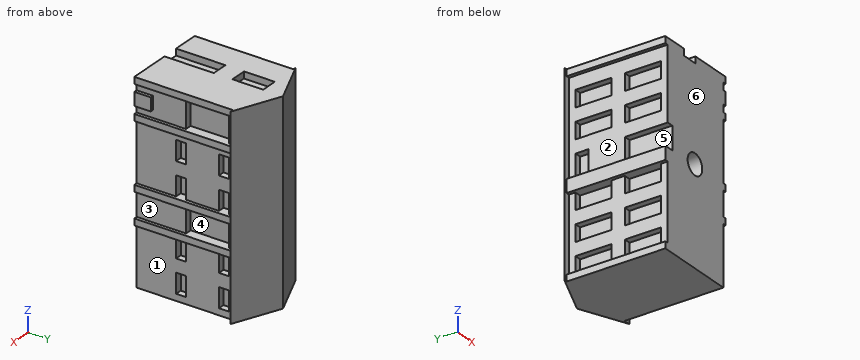
```python
from build123d import *

# Parameters (mm, degrees)
SALIENTE_EXTRUIR1_DEPTH = 30
CROQUIS2_W              = 1
CROQUIS2_H              = 15
SALIENTE_EXTRUIR2_DEPTH = 0.5
CROQUIS3_W              = 1
CROQUIS3_H              = 15
SALIENTE_EXTRUIR3_DEPTH = 0.5
CROQUIS3_3_W            = 3
CROQUIS3_3_H            = 1.5
CROQUIS3_3_W_2          = 3.754100145
CROQUIS3_3_H_2          = 6.5
CROQUIS3_3_W_3          = 4.245899855
CORTAR_EXTRUIR1_DEPTH   = 1
CROQUIS3_4_W            = 2
CROQUIS3_4_H            = 2.5
SALIENTE_EXTRUIR4_DEPTH = 0.5
CROQUIS7_W              = 1
CROQUIS7_H              = 15
SALIENTE_EXTRUIR5_DEPTH = 0.5
CROQUIS8_W              = 2.5
CROQUIS8_H              = 7.5
CROQUIS8_H_2            = 4.684108695
CORTAR_EXTRUIR2_DEPTH   = 1
CROQUIS10_W             = 1
CROQUIS10_H             = 15
CROQUIS10_W_2           = 2
SALIENTE_EXTRUIR6_DEPTH = 0.5
CROQUIS11_W             = 2.5
CROQUIS11_H             = 5.5
CORTAR_EXTRUIR3_DEPTH   = 1
CROQUIS12_W             = 3.5
CROQUIS12_H             = 6.5
CROQUIS12_H_2           = 2
CROQUIS12_W_2           = 2.5
CROQUIS12_H_3           = 5.5
CORTAR_EXTRUIR4_DEPTH   = 1
CROQUIS13_R             = 1.575
CORTAR_EXTRUIR5_DEPTH   = 2.5


with BuildPart() as part:
    # Croquis1 → Saliente-Extruir1 (new body)
    with BuildSketch(Plane.XY):
        Polygon((-6, -7.5), (6, -7.5), (6, 7.5), (7, 7.5), (0, 10.5), (-7, 7.5), (-6, 7.5), align=None)
    extrude(amount=SALIENTE_EXTRUIR1_DEPTH)

    # Croquis2 → Saliente-Extruir2 (add)
    with BuildSketch(Plane(origin=(6, 0, 0), x_dir=(0, 0, -1), z_dir=(1, 0, 0))):
        with Locations((-29.5, 0)):
            Rectangle(CROQUIS2_W, CROQUIS2_H)
        with Locations((-24.254100145, 0)):
            Rectangle(CROQUIS2_W, CROQUIS2_H)
    extrude(amount=SALIENTE_EXTRUIR2_DEPTH)

    # Croquis3 → Saliente-Extruir3 (add)
    with BuildSketch(Plane(origin=(6, 0, 0), x_dir=(0, 0, -1), z_dir=(1, 0, 0))):
        with Locations((-14.254100145, 0)):
            Rectangle(CROQUIS3_W, CROQUIS3_H)
        with Locations((-9.5, 0)):
            Rectangle(CROQUIS3_W, CROQUIS3_H)
    extrude(amount=SALIENTE_EXTRUIR3_DEPTH)

    # Croquis3_3 → Cortar-Extruir1 (cut)
    with BuildSketch(Plane(origin=(6, 0, 0), x_dir=(0, 0, -1), z_dir=(1, 0, 0))):
        with Locations((-21.254100145, 5.75)):
            Rectangle(CROQUIS3_3_W, CROQUIS3_3_H)
        with Locations((-16.254100145, 5.75)):
            Rectangle(CROQUIS3_3_W, CROQUIS3_3_H)
        with Locations((-16.254100145, -0.75)):
            Rectangle(CROQUIS3_3_W, CROQUIS3_3_H)
        with Locations((-21.254100145, -0.75)):
            Rectangle(CROQUIS3_3_W, CROQUIS3_3_H)
        with Locations((-7.5, -0.75)):
            Rectangle(CROQUIS3_3_W, CROQUIS3_3_H)
        with Locations((-2.5, -0.75)):
            Rectangle(CROQUIS3_3_W, CROQUIS3_3_H)
        with Locations((-11.877050073, 3.25)):
            Rectangle(CROQUIS3_3_W_2, CROQUIS3_3_H_2)
        with Locations((-7.5, 5.75)):
            Rectangle(CROQUIS3_3_W, CROQUIS3_3_H)
        with Locations((-2.5, 5.75)):
            Rectangle(CROQUIS3_3_W, CROQUIS3_3_H)
        with Locations((-26.877050073, 3.25)):
            Rectangle(CROQUIS3_3_W_3, CROQUIS3_3_H_2)
    extrude(amount=-CORTAR_EXTRUIR1_DEPTH, mode=Mode.SUBTRACT)

    # Croquis3_4 → Saliente-Extruir4 (add)
    with BuildSketch(Plane(origin=(6, 0, 0), x_dir=(0, 0, -1), z_dir=(1, 0, 0))):
        with Locations((-26.877050072, -6.25)):
            Rectangle(CROQUIS3_4_W, CROQUIS3_4_H)
    extrude(amount=SALIENTE_EXTRUIR4_DEPTH)

    # Croquis7 → Saliente-Extruir5 (add)
    with BuildSketch(Plane.ZY.offset(6)):
        with Locations((29.5, 0)):
            Rectangle(CROQUIS7_W, CROQUIS7_H)
    extrude(amount=SALIENTE_EXTRUIR5_DEPTH)

    # Croquis8 → Cortar-Extruir2 (cut)
    with BuildSketch(Plane.XY.offset(30)):
        with Locations((-1.25, -3.75)):
            Rectangle(CROQUIS8_W, CROQUIS8_H)
        with Locations((-1.25, 5.157945653)):
            Rectangle(CROQUIS8_W, CROQUIS8_H_2)
    extrude(amount=-CORTAR_EXTRUIR2_DEPTH, mode=Mode.SUBTRACT)

    # Croquis10 → Saliente-Extruir6 (add)
    with BuildSketch(Plane.ZY.offset(6)):
        with Locations((0.5, 0)):
            Rectangle(CROQUIS10_W, CROQUIS10_H)
        with Locations((13.5, 0)):
            Rectangle(CROQUIS10_W_2, CROQUIS10_H)
    extrude(amount=SALIENTE_EXTRUIR6_DEPTH)

    # Croquis11 → Cortar-Extruir3 (cut)
    with BuildSketch(Plane.ZY.offset(6)):
        with Locations((6.75, 3.75)):
            Rectangle(CROQUIS11_W, CROQUIS11_H)
        with Locations((2.25, 3.75)):
            Rectangle(CROQUIS11_W, CROQUIS11_H)
        with Locations((11.25, 3.75)):
            Rectangle(CROQUIS11_W, CROQUIS11_H)
        with Locations((6.75, -3.75)):
            Rectangle(CROQUIS11_W, CROQUIS11_H)
        with Locations((11.25, -3.75)):
            Rectangle(CROQUIS11_W, CROQUIS11_H)
        with Locations((2.25, -3.75)):
            Rectangle(CROQUIS11_W, CROQUIS11_H)
    extrude(amount=-CORTAR_EXTRUIR3_DEPTH, mode=Mode.SUBTRACT)

    # Croquis12 → Cortar-Extruir4 (cut)
    with BuildSketch(Plane.ZY.offset(6)):
        with Locations((16.25, -4.25)):
            Rectangle(CROQUIS12_W, CROQUIS12_H)
        with Locations((16.25, 5.5)):
            Rectangle(CROQUIS12_W, CROQUIS12_H_2)
        with Locations((21.25, 3.75)):
            Rectangle(CROQUIS12_W_2, CROQUIS12_H_3)
        with Locations((25.75, 3.75)):
            Rectangle(CROQUIS12_W_2, CROQUIS12_H_3)
        with Locations((21.25, -3.75)):
            Rectangle(CROQUIS12_W_2, CROQUIS12_H_3)
        with Locations((25.75, -3.75)):
            Rectangle(CROQUIS12_W_2, CROQUIS12_H_3)
    extrude(amount=-CORTAR_EXTRUIR4_DEPTH, mode=Mode.SUBTRACT)

    # Croquis13 → Cortar-Extruir5 (cut)
    with BuildSketch(Plane.XZ.offset(7.5)):
        with Locations(Location((-0.12745098, 14.705882353, 0), (0, 0, 270))):
            Circle(CROQUIS13_R)
    extrude(amount=-CORTAR_EXTRUIR5_DEPTH, mode=Mode.SUBTRACT)


solid = part.part
```
Source: CAD feature listing. Evaluate the final solid. Frame: model axes, mm. Face numbers are marked on the shaded views. A direction names the side the tool comes from. Round coordinates to 2 decimals unless told otherwise and drop trailing zeros. Order: outer loops, then holes, each group sorted by start corner. A loop starts at its lowest first (then second) coordinate and runs counter-clockwise, first axis right, second up. Notation, with made-up numbers: (77, 61.5) -> (99, 61.5) arc R20 cw to (99, 91.5) -> close; hole circle Ø5 at (-27, 43). An arc over 180 degrees is marked (long way). Use CSV: the item, a comma, the result in double quotes.
(1) Pull-direction query (Y, two-part tool) for the marked faces 4, 5 and 6; classes: +Y half, -Y half, draft (parallel to the pull), parting line (faces both ways), or undercut.
Report:
face 4,"undercut"
face 5,"draft"
face 6,"-Y half"
(2) Access query for the marked faces 1, 2 and 3. Directions: +Z, -Z, +X, -X, +Y, -Y. A direction counts if a zero-diameter tool reaches every point of the face in a straight line with its end or side. Return the directions, or none.
Report:
face 1,"-Z, +X, -Y"
face 2,"-X, -Y"
face 3,"+X, -Y"
(3) Section A-A on z = 11.25. Return the cut outline in (x, y), and give its area (4 significant figures).
Report:
outline,"(-7, 7.5) -> (-6, 7.5) -> (-6, 6.5) -> (-5, 6.5) -> (-5, 1) -> (-6, 1) -> (-6, -1) -> (-5, -1) -> (-5, -6.5) -> (-6, -6.5) -> (-6, -7.5) -> (6, -7.5) -> (6, 0) -> (5, 0) -> (5, 6.5) -> (6, 6.5) -> (6, 7.5) -> (7, 7.5) -> (0, 10.5) -> close"
area,"183.5 mm^2"
(4) First-contact query: pin 1 Ø1.9 at (y, z) = (-5.5, 12.5) entering from +X; pin 2 Ø0.8 at (y, z) = (-0.5, 3) entering from +X; pin 3 Ø0.5 at (x, z) = (-5.5, 2) entering from +Y. Flat tips, straight axial feed; report the tip coordinate or a pass-through.
Report:
pin 1,"x = 6"
pin 2,"x = 5"
pin 3,"y = 8.25"
(5) Section B-B on x = 1. Return the cut outline in (y, z), and give its area (3 significant figures).
Report:
outline,"(-7.5, 0) -> (10.07, 0) -> (10.07, 30) -> (-7.5, 30) -> (-7.5, 15.81) -> (-5, 15.81) -> (-5, 13.61) -> (-7.5, 13.61) -> close"
area,"522 mm^2"
(6) Section D-D on z = 19. Return the cut outline in (x, y), and give its area (3 significant figures).
Report:
outline,"(-7, 7.5) -> (-6, 7.5) -> (-6, -7.5) -> (6, -7.5) -> (6, 7.5) -> (7, 7.5) -> (0, 10.5) -> close"
area,"201 mm^2"
(7) Section C-C on y = 8.75. Return the cut outline in (x, z), and give its area (3 significant figures).
Report:
outline,"(-4.08, 0) -> (4.08, 0) -> (4.08, 30) -> (-4.08, 30) -> close"
area,"245 mm^2"
(8) Ray query, L1, parallel to Y at x = 5.5, z = 20; L2, parallel to Y at x = -5.75, z = 21.5; L3, parallel to X at y = 2, z = 13.5. Return the intervals inside material, ascending.
Report:
L1,"-7.5 to -1.5, 0 to 5, 6.5 to 8.14"
L2,"-7.5 to -6.5, -1 to 1, 6.5 to 8.04"
L3,"-6.5 to 5"
